```python
from build123d import *

# Parameters (mm, degrees)
BOX007_W          = 2.42
BOX007_H          = 1.69
BOX007_DEPTH      = 55
BOX008_W          = 2.42
BOX008_H          = 1.69
BOX008_DEPTH      = 55
CYLINDER002_R     = 0.9
CYLINDER002_DEPTH = 55
EXTRUDE011_DEPTH  = 53
FILLET_R          = 0.5


with BuildPart() as obj1:
    # Box007 → Box007 (new body)
    with BuildSketch(Plane(origin=(-3.63, 8.809483, 0), x_dir=(1, 0, 0), z_dir=(0, 0, 1))):
        with Locations((1.21, 0.845)):
            Rectangle(BOX007_W, BOX007_H)
    extrude(amount=BOX007_DEPTH)


with BuildPart() as cubo_der001:
    # Box008 → Box008 (new body)
    with BuildSketch(Plane(origin=(1.21, 8.809483, 0), x_dir=(1, 0, 0), z_dir=(0, 0, 1))):
        with Locations((1.21, 0.845)):
            Rectangle(BOX008_W, BOX008_H)
    extrude(amount=BOX008_DEPTH)


with BuildPart() as cilindro001:
    # Cylinder002 → Cylinder002 (new body)
    with BuildSketch(Plane(origin=(0, 11.9, 0), x_dir=(1, 0, 0), z_dir=(0, 0, 1))):
        Circle(CYLINDER002_R)
    extrude(amount=CYLINDER002_DEPTH)


with BuildPart() as obj2:
    # Sketch011 → Extrude011 (new body)
    with BuildSketch(Plane(origin=(0, -0.2, 0), x_dir=(1, 0, 0), z_dir=(0, 0, 1))):
        with BuildLine():
            ThreePointArc((-3.52341, 11.59655), (0, 8.899483), (3.52341, 11.59655))
            ThreePointArc((3.52341, 11.59655), (0, 12.12), (-3.52341, 11.59655))
        make_face()
    extrude(amount=EXTRUDE011_DEPTH)

    # Cut007: cut Cilindro001
    add(cilindro001.part, mode=Mode.SUBTRACT)

    # Cut008: cut Cubo der001
    add(cubo_der001.part, mode=Mode.SUBTRACT)

    # Cut009: cut obj1
    add(obj1.part, mode=Mode.SUBTRACT)

    # Fillet
    fillet_edges = [obj2.edges().sort_by_distance(p)[0] for p in [
        (-3.146427, 10.499483, 26.5),
        (-3.52341, 11.39655, 26.5),
        (-1.21, 10.499483, 26.5),
        (-0.899899, 11.886545, 26.5),
        (0.899899, 11.886545, 26.5),
        (3.52341, 11.39655, 26.5),
        (3.146427, 10.499483, 26.5),
        (1.21, 10.499483, 26.5),
        (1.21, 8.90588, 26.5),
        (-1.21, 8.90588, 26.5),
    ]]
    fillet(fillet_edges, radius=FILLET_R)


solid = obj2.part
```
Can you work these out from the model? Positions are in its coordinate system, mm. A direction names the side the tool comes from. Give positions to 0.01 mm unless a question says otherwise; leave off trailing zeros. Write each loop counter-clockwise with the first axis right and the second up, starting at its lowest first coordinate (ties: lowest second). Pieces come first, ordered by that corner, then holes. Notation, with made-up numbers: (88.25, 42.25) - (92.25, 42.25) arc R11 ccw to (92.25, 48.25) - close; hole circle Ø8 at (-4, 11.25). An arc over 180 degrees is marked (long way). Write item = value, one per line. Start each with the question number.
1. For pin 1 (0.9 mm diameter, centred on x = -2, z = 23.5, fed in from -Y); pin 2 (0.8 mm diameter, centred on y = 9.5, z = 23, fed in from +X); pin 3 (1 mm diameter, centred on y = 9.5, z = 35, fed in from -X), each with a flat end and sliding along its axis, tell me the tip position at first contact or that it passes through.
2. Please list where these lines run through material, in increasing order: line 1 (X direction, y = 9.6, z = 41.5); line 2 (X direction, y = 11.1, z = 9.5); line 3 (Y direction, x = -1.5, z = 21).
3. Thinking about a two-plate mould opening in X: for faces 1 (the face through (0, 11, 26)), 2 (the face through (-2, 10.499, 26)), 3 (the face through (0, 8.7, 26.1)), which applies, released by +X, released by -X, zero draft, split by the parting line, or undercut?
4. On a 3-axis mill with a long thin cutter (end or side, diameter ignored), from which of +Z, -Z, +X, -X, +Y, -Y can I reach the whole of each face in a straight line? I mean faces 4 (the face through (0, 10.6, 0)), 5 (the face through (2, 10.499, 26)). Say none if no direction works.
5. Imagine slicing it at A-A (x = 0). Please give me the cut outline in (y, z).
Worked answers:
q1.pin_1 = 10.47
q1.pin_2 = 1.21
q1.pin_3 = -1.21
q2.line_1 = -1.21 to 1.21
q2.line_2 = -3.37 to -0.41, 0.41 to 3.37
q2.line_3 = 10.45 to 11.83
q3.face_1 = undercut
q3.face_2 = zero draft
q3.face_3 = split by the parting line
q4.face_4 = -Z, +X, -X, +Y, -Y
q4.face_5 = +Z, -Z, +X, -Y
q5.outline = (8.7, 0) - (11, 0) - (11, 53) - (8.7, 53) - close
